from build123d import *

# Parameters (mm, degrees)
D52_D29_5_8_2_R                    = 26
D52_D29_5_8_2_R_2                  = 14.75
D52_D29_5_8_DEPTH                  = 8
D10_D24_8_2_R                      = 12
D10_D24_8_2_R_2                    = 5
D10_D24_8_DEPTH                    = 8
F_6XD3_4_D6_5_3_3_PCD42_AT_2_COUNT = 2
F_6XD3_4_D6_5_3_3_PCD42_AT_2_PITCH = 21
F_6XD3_4_D6_5_3_3_PCD42_AT_3_COUNT = 2
F_6XD3_4_D6_5_3_3_PCD42_AT_3_PITCH = 36.373066959
F_6XD3_4_D6_5_3_3_PCD42_AT_4_COUNT = 2
F_6XD3_4_D6_5_3_3_PCD42_AT_4_PITCH = 42
F_6XD3_4_D6_5_3_3_PCD42_AT_5_COUNT = 2
F_6XD3_4_D6_5_3_3_PCD42_AT_5_PITCH = 36.373066959
F_6XD3_4_D6_5_3_3_PCD42_AT_6_COUNT = 2
F_6XD3_4_D6_5_3_3_PCD42_AT_6_PITCH = 21
SKETCH_6_W                         = 1.25
SKETCH_6_H                         = 8
F_4XM3X0_5_PCD16_AT_2_COUNT        = 2
F_4XM3X0_5_PCD16_AT_2_PITCH        = 11.313708499
F_4XM3X0_5_PCD16_AT_3_COUNT        = 2
F_4XM3X0_5_PCD16_AT_3_PITCH        = 16
F_4XM3X0_5_PCD16_AT_4_COUNT        = 2
F_4XM3X0_5_PCD16_AT_4_PITCH        = 11.313708499
EXTRUDE_START                      = 7.25
SKETCH_2072_R                      = 14.7
SKETCH_2072_R_2                    = 12.08
EXTRUDE_2083_DEPTH                 = 0.55
EXTRUDE_START_2                    = 0.2
SKETCH_2120_R                      = 14.7
SKETCH_2120_R_2                    = 12.08
EXTRUDE_2131_DEPTH                 = 0.55


with BuildPart() as part:
    # D52__D29.5__8 2 → D52__D29.5__8 (new body)
    with BuildSketch(Plane.XY):
        Circle(D52_D29_5_8_2_R)
        Circle(D52_D29_5_8_2_R_2, mode=Mode.SUBTRACT)
    extrude(amount=D52_D29_5_8_DEPTH)

    # 草图4 → 外圈_6xD3.4通孔_D6.5沉孔深3.3_PCD42 (revolve, cut)
    with BuildSketch(Plane(origin=(18.186533479, 10.5, 8), x_dir=(0, -1, 0), z_dir=(1, 0, 0))):
        Polygon((0, 0), (0, 8), (1.7, 8), (1.7, 3.3), (3.25, 3.3), (3.25, 0), align=None)
    f_6xd3_4_d6_5_3_3_pcd42 = revolve(axis=Axis((18.186533479, 10.5, 14.35), (0, 0, -1)), mode=Mode.SUBTRACT)

    # 外圈_6xD3.4通孔_D6.5沉孔深3.3_PCD42 at 2: 外圈_6xD3.4通孔_D6.5沉孔深3.3_PCD42 ×2
    with Locations(*[(0, -i * F_6XD3_4_D6_5_3_3_PCD42_AT_2_PITCH, 0) for i in range(1, F_6XD3_4_D6_5_3_3_PCD42_AT_2_COUNT)]):
        add(f_6xd3_4_d6_5_3_3_pcd42, mode=Mode.SUBTRACT)

    # 外圈_6xD3.4通孔_D6.5沉孔深3.3_PCD42 at 3: 外圈_6xD3.4通孔_D6.5沉孔深3.3_PCD42 ×2
    with Locations(*[Vector(-0.5000000000000001, -0.8660254037844386, 0) * (i * F_6XD3_4_D6_5_3_3_PCD42_AT_3_PITCH) for i in range(1, F_6XD3_4_D6_5_3_3_PCD42_AT_3_COUNT)]):
        add(f_6xd3_4_d6_5_3_3_pcd42, mode=Mode.SUBTRACT)

    # 外圈_6xD3.4通孔_D6.5沉孔深3.3_PCD42 at 4: 外圈_6xD3.4通孔_D6.5沉孔深3.3_PCD42 ×2
    with Locations(*[Vector(-0.8660254037844387, -0.49999999999999983, 0) * (i * F_6XD3_4_D6_5_3_3_PCD42_AT_4_PITCH) for i in range(1, F_6XD3_4_D6_5_3_3_PCD42_AT_4_COUNT)]):
        add(f_6xd3_4_d6_5_3_3_pcd42, mode=Mode.SUBTRACT)

    # 外圈_6xD3.4通孔_D6.5沉孔深3.3_PCD42 at 5: 外圈_6xD3.4通孔_D6.5沉孔深3.3_PCD42 ×2
    with Locations(*[(-i * F_6XD3_4_D6_5_3_3_PCD42_AT_5_PITCH, 0, 0) for i in range(1, F_6XD3_4_D6_5_3_3_PCD42_AT_5_COUNT)]):
        add(f_6xd3_4_d6_5_3_3_pcd42, mode=Mode.SUBTRACT)

    # 外圈_6xD3.4通孔_D6.5沉孔深3.3_PCD42 at 6: 外圈_6xD3.4通孔_D6.5沉孔深3.3_PCD42 ×2
    with Locations(*[Vector(-0.8660254037844387, 0.5, 0) * (i * F_6XD3_4_D6_5_3_3_PCD42_AT_6_PITCH) for i in range(1, F_6XD3_4_D6_5_3_3_PCD42_AT_6_COUNT)]):
        add(f_6xd3_4_d6_5_3_3_pcd42, mode=Mode.SUBTRACT)


with BuildPart() as body_2:
    # D10__D24__8 2 → D10__D24__8 (new body)
    with BuildSketch(Plane.XY):
        Circle(D10_D24_8_2_R)
        Circle(D10_D24_8_2_R_2, mode=Mode.SUBTRACT)
    extrude(amount=D10_D24_8_DEPTH)

    # 草图6 → 内圈_4xM3x0.5通螺纹_PCD16 (revolve, cut)
    with BuildSketch(Plane(origin=(5.656854249, -5.656854249, 8), x_dir=(0, -1, 0), z_dir=(1, 0, 0))):
        with Locations((0.625, 4)):
            Rectangle(SKETCH_6_W, SKETCH_6_H)
    f_4xm3x0_5_pcd16 = revolve(axis=Axis((5.656854249, -5.656854249, 14.35), (0, 0, -1)), mode=Mode.SUBTRACT)

    # 内圈_4xM3x0.5通螺纹_PCD16 at 2: 内圈_4xM3x0.5通螺纹_PCD16 ×2
    with Locations(*[(-i * F_4XM3X0_5_PCD16_AT_2_PITCH, 0, 0) for i in range(1, F_4XM3X0_5_PCD16_AT_2_COUNT)]):
        add(f_4xm3x0_5_pcd16, mode=Mode.SUBTRACT)

    # 内圈_4xM3x0.5通螺纹_PCD16 at 3: 内圈_4xM3x0.5通螺纹_PCD16 ×2
    with Locations(*[Vector(-0.7071067811865475, 0.7071067811865477, 0) * (i * F_4XM3X0_5_PCD16_AT_3_PITCH) for i in range(1, F_4XM3X0_5_PCD16_AT_3_COUNT)]):
        add(f_4xm3x0_5_pcd16, mode=Mode.SUBTRACT)

    # 内圈_4xM3x0.5通螺纹_PCD16 at 4: 内圈_4xM3x0.5通螺纹_PCD16 ×2
    with Locations(*[(0, i * F_4XM3X0_5_PCD16_AT_4_PITCH, 0) for i in range(1, F_4XM3X0_5_PCD16_AT_4_COUNT)]):
        add(f_4xm3x0_5_pcd16, mode=Mode.SUBTRACT)


with BuildPart() as body_3:
    # Sketch 2072 → Extrude 2083 (new body)
    with BuildSketch(Plane.XY.offset(EXTRUDE_START)):
        Circle(SKETCH_2072_R)
        Circle(SKETCH_2072_R_2, mode=Mode.SUBTRACT)
    extrude(amount=EXTRUDE_2083_DEPTH)


with BuildPart() as body_4:
    # Sketch 2120 → Extrude 2131 (new body)
    with BuildSketch(Plane.XY.offset(EXTRUDE_START_2)):
        Circle(SKETCH_2120_R)
        Circle(SKETCH_2120_R_2, mode=Mode.SUBTRACT)
    extrude(amount=EXTRUDE_2131_DEPTH)


solid = body_2.part
Source: CAD feature listing. Evaluate the final solid. Frame: model axes, mm. Coordinates: 2 decimals unless noted, no trailing zeros. Order: outer loops, then holes, each group sorted by start corner. A loop starts at its lowest first (then second) coordinate and runs counter-clockwise, first axis right, second up. Notation, with made-up numbers: M 73.25,52 L 94.25,52 A15 ccw 94.25,77 Z; hole C 85.25,55.25 d7. An arc over 180 degrees is marked long. Write each question's results on one line, items separated by ' | '. Start each with the question number.
Item 1: Draft query along X for faces 1 (the face through (5.2, 0.2, 8)), 2 (the face through (-5.712, -4.408, 3.944)), 3 (the face through (-11.99, 0.53, 3.94)). Return one class per face: pulls with the +X half, pulls with the -X half, needs draft (parallel to the pull), parting line crosses it, or undercut.
Item 2: Line query: probe 1 along Y at (x, z) = (0, 4.75); probe 2 along X at (y, z) = (5.5, 1); probe 3 along X at (y, z) = (5.25, 2.5). Output: solid intervals per line, ascending.
Item 3: Cut plane D-D (x = -8). Return loops of the section in (y, z), and give its area (3 significant figures).
Item 4: Cut plane A-A (x = 0). Return loops of the section in (y, z), and give its area (3 significant figures).
Item 5: First-contact query: pin 1 Ø1 at (y, z) = (-6.5, 3.5) entering from -X; pin 2 Ø1.5 at (y, z) = (-8.5, 6) entering from -X; pin 3 Ø6 at (x, y) = (0, 0) entering from -Z; pin 4 Ø4 at (y, z) = (5.5, 6) entering from +X. Flat tips, straight axial feed; report the tip coordinate or a pass-through.
Item 6: Cut plane B-B (y = -3.75). Return loops of the section in (x, z).
Item 7: Cut plane C-C (z = 1.25). Return loops of the section in (x, y).
Checked values:
1) face 1: needs draft | face 2: undercut | face 3: parting line crosses it
2) probe 1: y = -12 to -5, 5 to 12 | probe 2: x = -10.67 to -6.9, -4.42 to 4.42, 6.9 to 10.67 | probe 3: x = -10.79 to -6.84, -4.47 to 4.47, 6.84 to 10.79
3) outline: M -8.94,0 L 8.94,0 L 8.94,8 L -8.94,8 Z | area: 143 mm2
4) outline: M -12,0 L -5,0 L -5,8 L -12,8 Z; M 5,0 L 12,0 L 12,8 L 5,8 Z | area: 112 mm2
5) pin 1: stops at x = -10.39 | pin 2: stops at x = -9.16 | pin 3: passes through | pin 4: stops at x = 11.48
6) outline: M -11.4,0 L -3.31,0 L -3.31,8 L -11.4,8 Z; M 3.31,0 L 11.4,0 L 11.4,8 L 3.31,8 Z
7) outline: C 0,0 d24; hole C -5.66,-5.66 d2.5; hole C -5.66,5.66 d2.5; hole C 0,0 d10; hole C 5.66,-5.66 d2.5; hole C 5.66,5.66 d2.5
